Input: dimensioned drawing with shaded views. Units: mm. Origin: part minimum x, y, z. A direction names the side the tool comes from. Coordinates: 2 decimals unless noted, no trailing zeros. Write each loop counter-clockwise with the first axis right and the second up, starting at its lowest first coordinate (ties: lowest second). Pieces come first, ordered by that corner, then holes. Notation, with made-up numbers: M 46.25,-17.75 L 64.25,-17.75 A31 ccw 64.25,10.25 Z; hole C 23.5,61 d1. An arc over 180 degrees is marked long. Write each question's results on one line, items separated by ' | '. Start each with the question number.
1. First-contact query: pin 1 (2 mm diameter, centred on x = 2, z = 13.5, fed in from +Y); pin 2 (2 mm diameter, centred on y = 2, z = 40, fed in from -X). Flat tips, straight axial feed; report the tip coordinate or a pass-through.
2. Section query C-C, the plane z = 8. Output: boundary loops of the cut face in (x, y).
3. Ray query, probe 1 along X at (y, z) = (5.5, 1.5); probe 2 along Z at (x, y) = (2.5, 2.5); probe 3 along X at (y, z) = (5.25, 27.5). Return the intervals inside material, ascending.
4. Section query A-A, the plane y = 8.5. Output: boundary loops of the cut face in (x, z).
5. Set-up query: the marked faces 1 and 2. Return all of +Z, -Z, +X, -X, +Y, -Y with unobstructed straight access to the full face (end or side cutting, diameter ignored); none if empty.
6. Section query B-B, the plane z = 32. Output: boundary loops of the cut face in (x, y), and give its area (3 significant figures).
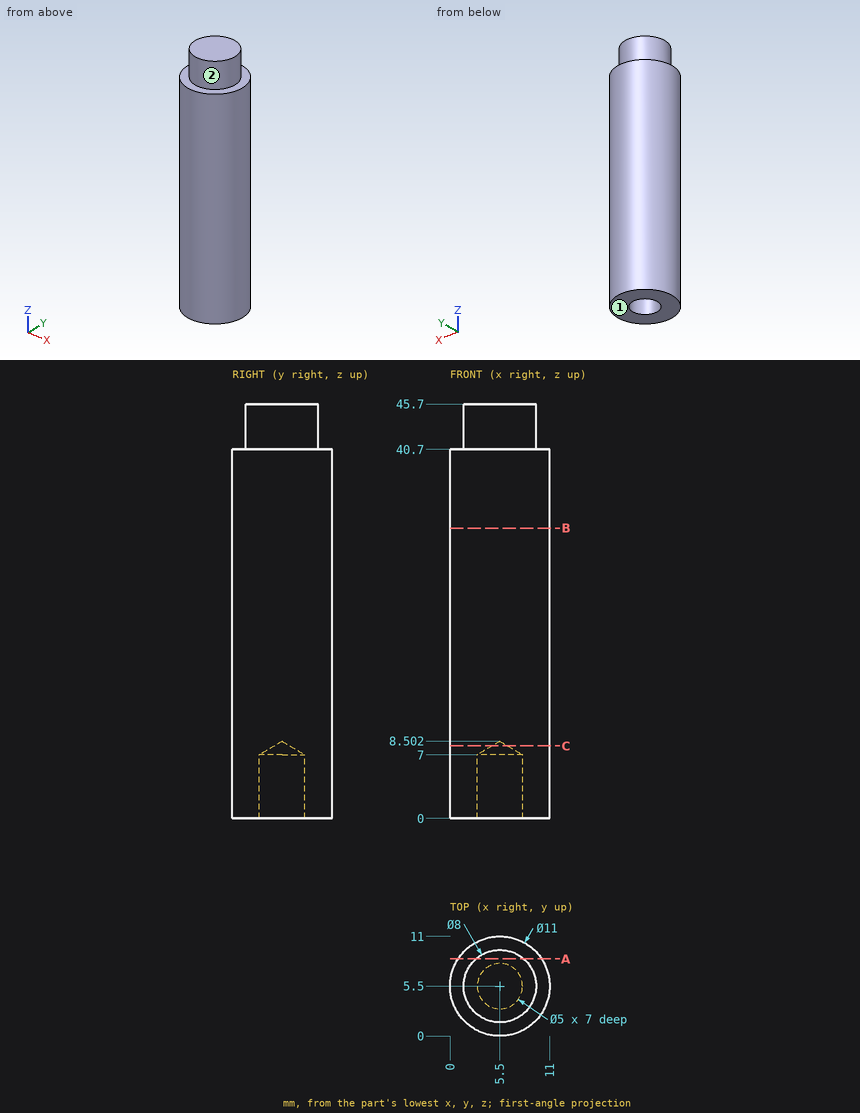
Answer:
1) pin 1: y = 10.4 | pin 2: x = 0.6
2) outline: C 5.5,5.5 d11; hole C 5.5,5.5 d1.67
3) probe 1: 0 to 3, 8 to 11 | probe 2: 0 to 40.7 | probe 3: 0.01 to 10.99
4) outline: M 0.89,0 L 10.11,0 L 10.11,40.7 L 8.15,40.7 L 8.15,45.7 L 2.85,45.7 L 2.85,40.7 L 0.89,40.7 Z
5) face 1: -Z, +X, -X, +Y, -Y | face 2: +Z
6) outline: C 5.5,5.5 d11 | area: 95.0 mm^2
